Design review of the part built by this model. Coordinates are the model's own, in mm. A direction names the side the tool comes from. Round coordinates to 2 decimals unless told otherwise and drop trailing zeros. Order: outer loops, then holes, each group sorted by start corner. A loop starts at its lowest first (then second) coordinate and runs counter-clockwise, first axis right, second up. Notation, with made-up numbers: (60, -1.75) - (95, -1.75) arc R12 ccw to (95, 21.25) - close; hole circle Ø1 at (0.25, 83). An arc over 180 degrees is marked (long way). Answer as a JSON object with one key per item and string values. Group by question number.
from build123d import *

# Parameters (mm, degrees)
F0_W     = 8
F0_H     = 8
F1_DEPTH = 4
F2_R     = 4
F3_R     = 3.99999


# Not quite as in the source:
# - a fillet or chamfer is up to 0.001 mm smaller than in the source, because OpenCascade refuses the exact size


with BuildPart() as f1:
    # F0 (on Top) → F1 (new body)
    with BuildSketch(Plane.XY):
        Rectangle(F0_W, F0_H)
        with BuildLine():
            Line((-1.9619476116, -2), (-1.9619476116, 1))
            ThreePointArc((-1.9619476116, 1), (0.0380527829, 2.9999996055), (2.0380523884, 0.9999992109))
            Line((2.0380523884, 0.9999992109), (2.0380523884, -2))
            Line((2.0380523884, -2), (-1.9619476116, -2))
        make_face(mode=Mode.SUBTRACT)
    extrude(amount=F1_DEPTH)

    # F2
    f2_edges = [f1.edges().sort_by_distance(p)[0] for p in [
        (4, 4, 2),
    ]]
    fillet(f2_edges, radius=F2_R)

    # F3 (radius 4 in the source; OpenCascade refuses exactly that, so slightly less here)
    f3_edges = [f1.edges().sort_by_distance(p)[0] for p in [
        (-4, 4, 2),
    ]]
    fillet(f3_edges, radius=F3_R)


solid = f1.part
1. Take a section at A-A, the plane y = -1. Give the boundary of the cut face in (x, z).
2. Mouldability with a two-part tool opening along Y and no side actions: class faces 3 (the cylindrical face through (2.797, 2.859, 2.028)), 4 (the flat face through (0, -2, 2)), 5 (the flat face through (0, -3, 4)) as pulls with the +Y half, pulls with the -Y half, needs draft (parallel to the pull), parting line crosses it, or undercut.
3. Take a section at C-C, the plane x = -1.5. Give the boundary of the cut face in (y, z), then the cut area to 3 significant figures.
4. Clearance check with a flat-ended pin moving along its axis: P1, Ø1.5, axis at y = 2.5, z = 0.5, coming from the +X side. State where the tip first meets the part, or that it passes through.
5. To check wall thickness, follow line 1 (X direction, y = -0.5, z = 3.45); line 2 (Y direction, x = -1.5, z = 3.8); line 3 (Y direction, x = -1.25, z = 1.85). State the ranges of each line that lie inside material, in increasing order. Write a range as from..to.
6. Tool access review of faces 1 (the flat face through (-1.962, -1, 2)), 2 (the flat face through (0, -3, 0)): name each direction out of +Z, -Z, +X, -X, +Y, -Y from which nothing blocks a thin tool from reaching the whole face with its end or side.
7. Take a section at D-D, the plane x = -2.75. Give the boundary of the cut face in (y, z), then the cut area to 3 significant figures.
Response values:
{
 "1": {"outline": "(-4, 0) - (-1.96, 0) - (-1.96, 4) - (-4, 4) - close; (2.04, 0) - (4, 0) - (4, 4) - (2.04, 4) - close"},
 "2": {"face 3": "pulls with the +Y half", "face 4": "undercut", "face 5": "needs draft"},
 "3": {"outline": "(-4, 0) - (-2, 0) - (-2, 4) - (-4, 4) - close; (2.28, 0) - (3.71, 0) - (3.71, 4) - (2.28, 4) - close", "area": "13.7 mm2"},
 "4": {"P1": "x = 3.6"},
 "5": {"line 1": "-4..-1.96, 2.04..4", "line 2": "-4..-2, 2.28..3.71", "line 3": "-4..-2, 2.53..3.8"},
 "6": {"face 1": "+Z, -Z", "face 2": "-Z, +X, -X, +Y, -Y"},
 "7": {"outline": "(-4, 0) - (2.9, 0) - (2.9, 4) - (-4, 4) - close", "area": "27.6 mm2"}
}
